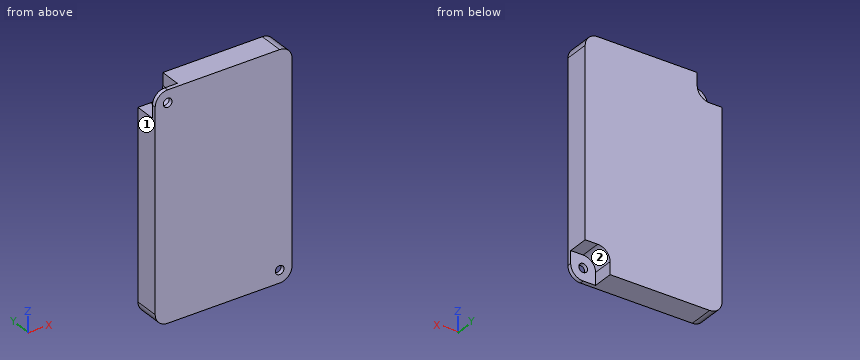
from build123d import *

# Parameters (mm, degrees)
SKETCH_1_R          = 1.75
EXTRUDE_1_DEPTH     = 10
SKETCH_2_R          = 1.75
CUT_EXTRUDE_2_DEPTH = 8.4


with BuildPart() as part:
    # 草图1 → 凸台-拉伸1 (new body)
    with BuildSketch(Plane(origin=(0, 0, 0), x_dir=(1, 0, 0), z_dir=(0, 1, 0))):
        with BuildLine():
            Line((-22.5, -45), (22.5, -45))
            ThreePointArc((22.5, -45), (26.035533906, -43.535533906), (27.5, -40))
            Line((27.5, -40), (27.5, 40))
            ThreePointArc((27.5, 40), (26.035533906, 43.535533906), (22.5, 45))
            Line((22.5, 45), (-22.5, 45))
            ThreePointArc((-22.5, 45), (-26.035533906, 43.535533906), (-27.5, 40))
            Line((-27.5, 40), (-27.5, -40))
            ThreePointArc((-27.5, -40), (-26.035533906, -43.535533906), (-22.5, -45))
        make_face()
        with Locations((-22.5, -40)):
            Circle(SKETCH_1_R, mode=Mode.SUBTRACT)
        with Locations((22.5, 40)):
            Circle(SKETCH_1_R, mode=Mode.SUBTRACT)
    extrude(amount=EXTRUDE_1_DEPTH)

    # 草图2 → 切除-拉伸2 (cut)
    with BuildSketch(Plane(origin=(0, 10, 0), x_dir=(1, 0, 0), z_dir=(0, 1, 0))):
        with BuildLine():
            Line((-27.5, -35), (-27.5, -40))
            ThreePointArc((-27.5, -40), (-26.035533906, -43.535533906), (-22.5, -45))
            Line((-22.5, -45), (-17.5, -45))
            Line((-17.5, -45), (-17.5, -40))
            ThreePointArc((-17.5, -40), (-18.964466094, -36.464466094), (-22.5, -35))
            Line((-22.5, -35), (-27.5, -35))
        make_face()
        with Locations((-22.5, -40)):
            Circle(SKETCH_2_R, mode=Mode.SUBTRACT)
        with BuildLine():
            Line((22.5, 45), (17.5, 45))
            Line((17.5, 45), (17.5, 40))
            ThreePointArc((17.5, 40), (18.964466094, 36.464466094), (22.5, 35))
            Line((22.5, 35), (27.5, 35))
            Line((27.5, 35), (27.5, 40))
            ThreePointArc((27.5, 40), (26.035533906, 43.535533906), (22.5, 45))
        make_face()
        with Locations((22.5, 40)):
            Circle(SKETCH_2_R, mode=Mode.SUBTRACT)
    extrude(amount=-CUT_EXTRUDE_2_DEPTH, mode=Mode.SUBTRACT)


solid = part.part
Geometry: final body of the model. Coordinates: model frame, mm. Face numbers are marked on the shaded views. A direction names the side the tool comes from. Coordinates: 2 decimals unless noted, no trailing zeros. Order: outer loops, then holes, each group sorted by start corner. A loop starts at its lowest first (then second) coordinate and runs counter-clockwise, first axis right, second up.
1) Section A-A (y = 5.5). Return loops of the section in (x, z).
Result sheet:
outline: (-27.5, -40) arc R5 ccw to (-22.5, -45) - (17.5, -45) - (17.5, -40) arc R5 cw to (22.5, -35) - (27.5, -35) - (27.5, 40) arc R5 ccw to (22.5, 45) - (-17.5, 45) - (-17.5, 40) arc R5 cw to (-22.5, 35) - (-27.5, 35) - close
2) Set-up query: the marked faces 1 and 2. Return all of +Z, -Z, +X, -X, +Y, -Y with unobstructed straight access to the full face (end or side cutting, diameter ignored); none if empty.
Result sheet:
face 1: +Z, -Z, -X, +Y, -Y
face 2: -Z, +X, +Y
3) First-contact query: P1, Ø4, axis at y = 5.5, z = -43, coming from the +X side; P2, Ø1.5, axis at y = 5.5, z = 43, coming from the -X side; P3, Ø2.5, axis at x = -24, y = 7.5, coming from the +Z side. Flat tips, straight axial feed; report the tip coordinate or a pass-through.
Result sheet:
P1: stops at x = 17.5
P2: stops at x = -17.5
P3: stops at z = 35
4) Ray query, probe 1 along X at (y, z) = (0.5, -40); probe 2 along Z at (x, y) = (22.5, 0.95); probe 3 along Z at (x, y) = (-22.5, 0.55). Return the intervals inside material, ascending.
Result sheet:
probe 1: x = -27.5 to 20.75, 24.25 to 27.5
probe 2: z = -45 to -41.75, -38.25 to 45
probe 3: z = -45 to 38.25, 41.75 to 45
